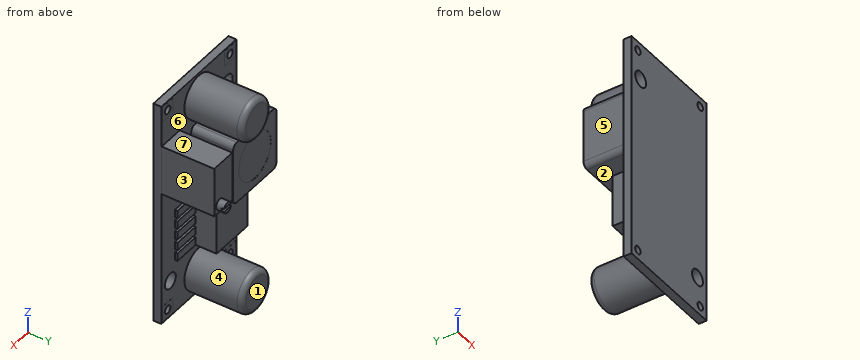
Autodesk Inventor part; units mm, degrees
ref_plane "YZ Plane" through (0, 0, 0) normal (1, 0, 0) x (0, 1, 0)
ref_plane "XZ Plane" through (0, 0, 0) normal (0, 1, 0) x (-1, 0, 0)
ref_plane "XY Plane" through (0, 0, 0) normal (0, 0, 1) x (1, 0, 0)
sketch "Sketch1" plane through (0, 0, 0) normal (0, 1, 0) x (-1, 0, 0)
  line L0 (-10.375, 21.675) -> (10.375, 21.675)
  line L1 (10.375, 21.675) -> (10.375, -21.675)
  line L2 (10.375, -21.675) -> (-10.375, -21.675)
  line L3 (-10.375, -21.675) -> (-10.375, 21.675)
  line L4 (-10.375, 21.675) -> (10.375, -21.675) construction
  line L5 (10.375, 21.675) -> (-10.375, -21.675) construction
  point P0 (0, 0)
  dimension "d0" = 20.75
  dimension "d1" = 43.35
extrude "Extrusion1" add sketch "Sketch1" along normal blind 1.5
sketch "Sketch2" plane through (0, 1.5, 0) normal (0, 1, 0) x (1, 0, 0)
  circle A0 centre (-8.625, -19.925) radius 0.75
  circle A1 centre (-8.625, 19.925) radius 0.75
  circle A2 centre (8.625, -19.925) radius 0.75
  circle A3 centre (8.625, 19.925) radius 0.75
  line L0 (-10.375, -21.675) -> (10.375, -21.675)
  line L1 (10.375, -21.675) -> (10.375, 21.675)
  line L2 (-10.375, 21.675) -> (-10.375, -21.675)
  line L3 (10.375, 21.675) -> (-10.375, 21.675)
  point P0 (0, 0)
  dimension "d4" = 1.5
  dimension "d5" = 1.5
  dimension "d6" = 1.5
  dimension "d7" = 1.5
  dimension "d8" = 1.75
  dimension "d9" = 1.75
  dimension "d10" = 1.75
  dimension "d11" = 1.75
  dimension "d12" = 1.75
  dimension "d13" = 1.75
  dimension "d14" = 1.75
  dimension "d15" = 1.75
extrude "Extrusion2" cut sketch "Sketch2" against normal up to next contours A0 | A1 | A2 | A3
sketch "Sketch3" plane through (0, 1.5, 0) normal (0, 1, 0) x (1, 0, 0)
  circle A0 centre (7.875, 14.675) radius 1.5
  circle A1 centre (-7.875, -14.675) radius 1.5
  line L0 (-10.375, 21.675) -> (-10.375, -21.675)
  line L1 (10.375, 21.675) -> (10.375, -21.675)
  line L2 (10.375, 21.675) -> (-10.375, 21.675)
  line L3 (-10.375, -21.675) -> (10.375, -21.675)
  point P0 (0, 0)
  dimension "d18" = 3
  dimension "d19" = 3
  dimension "d20" = 2.5
  dimension "d21" = 2.5
  dimension "d22" = 7
  dimension "d23" = 7
extrude "Extrusion3" cut sketch "Sketch3" against normal up to next contours A0 | A1
sketch "Sketch4" plane through (0, 1.5, 0) normal (0, 1, 0) x (1, 0, 0)
  line L0 (-7.125, -18.425) -> (-10.125, -18.425)
  line L1 (-10.125, -18.425) -> (-10.125, -21.425)
  line L2 (-10.125, -21.425) -> (-7.125, -21.425)
  line L3 (-7.125, -21.425) -> (-7.125, -18.425)
  circle A0 centre (-8.625, -19.925) radius 0.75
  line L4 (-7.125, -18.425) -> (-10.125, -21.425) construction
  line L5 (-10.125, -18.425) -> (-7.125, -21.425) construction
  line L6 (10.125, -21.425) -> (7.125, -21.425)
  line L7 (7.125, -21.425) -> (7.125, -18.425)
  line L8 (7.125, -18.425) -> (10.125, -18.425)
  line L9 (10.125, -18.425) -> (10.125, -21.425)
  circle A1 centre (8.625, -19.925) radius 0.75
  line L10 (10.125, -21.425) -> (7.125, -18.425) construction
  line L11 (7.125, -21.425) -> (10.125, -18.425) construction
  line L12 (7.125, 18.425) -> (10.125, 18.425)
  line L13 (10.125, 18.425) -> (10.125, 21.425)
  line L14 (10.125, 21.425) -> (7.125, 21.425)
  line L15 (7.125, 21.425) -> (7.125, 18.425)
  circle A2 centre (8.625, 19.925) radius 0.75
  line L16 (7.125, 18.425) -> (10.125, 21.425) construction
  line L17 (10.125, 18.425) -> (7.125, 21.425) construction
  line L18 (-10.125, 21.425) -> (-7.125, 21.425)
  line L19 (-7.125, 21.425) -> (-7.125, 18.425)
  line L20 (-7.125, 18.425) -> (-10.125, 18.425)
  line L21 (-10.125, 18.425) -> (-10.125, 21.425)
  circle A3 centre (-8.625, 19.925) radius 0.75
  line L22 (-10.125, 21.425) -> (-7.125, 18.425) construction
  line L23 (-7.125, 21.425) -> (-10.125, 18.425) construction
  circle A4 centre (-8.625, -19.925) radius 0.75
  circle A5 centre (8.625, -19.925) radius 0.75
  circle A6 centre (-8.625, 19.925) radius 0.75
  circle A7 centre (8.625, 19.925) radius 0.75
  point P0 (0, 0)
  dimension "d26" = 3
  dimension "d27" = 3
  dimension "d28" = 3
  dimension "d29" = 3
  dimension "d30" = 3
  dimension "d31" = 3
  dimension "d32" = 3
  dimension "d33" = 3
extrude "Extrusion4" add sketch "Sketch4" along normal blind 0.01
sketch "Sketch5" plane through (0, 1.5, 0) normal (0, 1, 0) x (1, 0, 0)
  circle A0 centre (0, 17.175) radius 4
  line L0 (10.375, 21.675) -> (-10.375, 21.675)
  point P0 (0, 0)
  dimension "d36" = 8
  dimension "d37" = 4.5
extrude "Extrusion5" add sketch "Sketch5" along normal blind 11
sketch "Sketch6" plane through (0, 1.5, 0) normal (0, 1, 0) x (1, 0, 0)
  circle A0 centre (0, -17.175) radius 4
  line L0 (-10.375, -21.675) -> (10.375, -21.675)
  point P0 (0, 0)
  dimension "d40" = 8
  dimension "d41" = 4.5
extrude "Extrusion6" add sketch "Sketch6" along normal blind 11
sketch "Sketch7" plane through (0, 1.5, 0) normal (0, 1, 0) x (1, 0, 0)
  line L0 (2.125, -12.175) -> (-9.875, -12.175)
  line L1 (-9.875, -12.175) -> (-9.875, -0.175)
  line L2 (-9.875, -0.175) -> (2.125, -0.175)
  line L3 (2.125, -0.175) -> (2.125, -12.175)
  line L4 (2.125, -12.175) -> (-9.875, -0.175) construction
  line L5 (-9.875, -12.175) -> (2.125, -0.175) construction
  line L6 (-10.375, 21.675) -> (-10.375, -21.675)
  circle A0 centre (0, -17.175) radius 4
  point P0 (0, 0)
  point P1 (-3.875, -6.175)
  dimension "d44" = 12
  dimension "d45" = 12
  dimension "d46" = 0.5
  dimension "d47" = 5
extrude "Extrusion7" add sketch "Sketch7" along normal blind 8 contours L0 L1 L2 L3
sketch "Sketch8" plane through (0, 9.5, 0) normal (0, 1, 0) x (1, 0, 0)
  line L0 (2.125, -12.175) -> (-9.875, -12.175)
  line L1 (-9.875, -12.175) -> (2.125, -0.175)
  circle A0 centre (-3.875, -6.175) radius 4.4338
  point P0 (0, 0)
extrude "Extrusion8" cut sketch "Sketch8" against normal blind 0.01
sketch "Sketch9" plane through (0, 1.5, 0) normal (0, 1, 0) x (1, 0, 0)
  line L0 (10.275, -13.675) -> (5.275, -13.675)
  line L1 (5.275, -13.675) -> (5.275, -4.175)
  line L2 (5.275, -4.175) -> (10.275, -4.175)
  line L3 (10.275, -4.175) -> (10.275, -13.675)
  line L4 (10.275, -13.675) -> (5.275, -4.175) construction
  line L5 (5.275, -13.675) -> (10.275, -4.175) construction
  line L6 (-10.375, -21.675) -> (10.375, -21.675)
  line L7 (10.375, 21.675) -> (10.375, -21.675)
  point P0 (0, 0)
  point P1 (7.775, -8.925)
  dimension "d52" = 5
  dimension "d53" = 9.5
  dimension "d54" = 8
  dimension "d55" = 0.1
extrude "Extrusion9" add sketch "Sketch9" along normal blind 10
sketch "Sketch10" plane through (0, 11.5, 0) normal (0, 1, 0) x (1, 0, 0)
  circle A0 centre (8.775, -5.675) radius 1
  line L0 (10.275, -4.175) -> (5.275, -4.175)
  line L1 (10.275, -13.675) -> (10.275, -4.175)
  point P0 (0, 0)
  dimension "d58" = 2
  dimension "d59" = 1.5
  dimension "d60" = 1.5
extrude "Extrusion10" add sketch "Sketch10" along normal blind 1.5
sketch "Sketch11" plane through (8.775, 13, 5.675) normal (0, 1, 0) x (1, 0, 0)
  line L0 (1.224, -0.2665) -> (-1.224, -0.2665)
  line L1 (-1.224, -0.2665) -> (-1.224, 0.2665)
  line L2 (-1.224, 0.2665) -> (1.224, 0.2665)
  line L3 (1.224, 0.2665) -> (1.224, -0.2665)
  line L4 (1.224, -0.2665) -> (-1.224, 0.2665) construction
  line L5 (-1.224, -0.2665) -> (1.224, 0.2665) construction
  point P0 (-8.775, 5.675)
  point P1 (0, 0)
extrude "Extrusion11" cut sketch "Sketch11" against normal blind 0.5
sketch "Sketch12" plane through (0, 1.5, 0) normal (0, 1, 0) x (1, 0, 0)
  line L0 (1.625, 1.325) -> (-6.875, 1.325)
  line L1 (-6.875, 1.325) -> (-6.875, 11.325)
  line L2 (-6.875, 11.325) -> (1.625, 11.325)
  line L3 (1.625, 11.325) -> (1.625, 1.325)
  line L4 (1.625, 1.325) -> (-6.875, 11.325) construction
  line L5 (-6.875, 1.325) -> (1.625, 11.325) construction
  line L6 (-10.375, 21.675) -> (-10.375, -21.675)
  line L7 (2.125, -0.175) -> (-9.875, -0.175)
  point P0 (0, 0)
  point P1 (-2.625, 6.325)
  dimension "d65" = 8.5
  dimension "d66" = 10
  dimension "d67" = 3.5
  dimension "d68" = 1.5
extrude "Extrusion12" add sketch "Sketch12" along normal blind 4.5
sketch "Sketch13" plane through (1.625, 1.5, -1.325) normal (1, 0, 0) x (0, 0, -1)
  line L0 (10, 0) -> (0, 0)
  line L1 (0, 0) -> (1.5, 0)
  line L2 (1.5, 0) -> (1.5, 0.5)
  line L3 (1.5, 0.5) -> (0, 0.5)
  line L4 (0, 0.5) -> (0, 0)
  line L5 (10, 0) -> (8.5, 0)
  line L6 (8.5, 0) -> (8.5, 0.5)
  line L7 (8.5, 0.5) -> (10, 0.5)
  line L8 (10, 0.5) -> (10, 0)
  line L9 (2.12, 0) -> (3.62, 0)
  line L10 (3.62, 0) -> (3.62, 0.5)
  line L11 (3.62, 0.5) -> (2.12, 0.5)
  line L12 (2.12, 0.5) -> (2.12, 0)
  line L13 (6.38, 0) -> (7.88, 0)
  line L14 (7.88, 0) -> (7.88, 0.5)
  line L15 (7.88, 0.5) -> (6.38, 0.5)
  line L16 (6.38, 0.5) -> (6.38, 0)
  line L17 (4.24, 0) -> (5.74, 0)
  line L18 (5.74, 0) -> (5.74, 0.5)
  line L19 (5.74, 0.5) -> (4.24, 0.5)
  line L20 (4.24, 0.5) -> (4.24, 0)
  point P0 (-1.325, -1.5)
  dimension "d71" = 1.5
  dimension "d72" = 0.5
  dimension "d73" = 1.5
  dimension "d74" = 0.5
  dimension "d75" = 1.5
  dimension "d76" = 1.5
  dimension "d77" = 0.5
  dimension "d78" = 0.62
  dimension "d79" = 0.62
  dimension "d80" = 1.5
  dimension "d81" = 0.62
extrude "Extrusion13" add sketch "Sketch13" along normal blind 5
fillet "Fillet1" radius 1 6 edges at (2.125, 5.5, 12.175) (2.125, 5.5, 0.175) (-9.875, 5.5, 12.175) (-9.875, 5.5, 0.175) (-4, 12.5, 17.175) (-4, 12.5, -17.175)
properties part number "pcb_with_elements"
Geometry check sheet. Reference: the model listing, model coordinates, mm. Face numbers are marked on the shaded views. A direction names the side the tool comes from. Give positions to 0.01 mm unless a question says otherwise; leave off trailing zeros. Loops run counter-clockwise (first coordinate to the right, second up) from the corner with the lowest first, then second, coordinate; pieces in that order, holes last. Notation, with made-up numbers: (81, 38) - (107, 38) arc R19 ccw to (107, 66) - close; hole circle Ø9 at (59, 81). An arc over 180 degrees is marked (long way). Use CSV: the item, a comma, the result in double quotes. Start each with the question number.
Q1. Scan lines: probe 1 along X at (y, z) = (5.5, 11) (3 decimals); probe 2 along Z at (x, y) = (1.5, 4.75) (3 decimals); probe 3 along X at (y, z) = (4.75, -3.5) (3 decimals). Record each from-to range of solid material in increasing order. Write a range as from..to.
Q2. Access from +Z, -Z, +X, -X, +Y, -Y to the whole of each face (thin tool, end or side, straight path). Record for the marked faces 1, 2, 3 and 4.
Q3. Go/stop test with flat-tipped pins: pin 1 Ø0.8 at (x, z) = (3.5, -10.5) entering from +Y; pin 2 Ø3 at (x, y) = (3.5, 11.5) entering from +Z; pin 3 Ø1.5 at (x, y) = (6.5, 9) entering from -Z (3 decimals). Record where each tip stops, or that it passes through.
Q4. Section check B-B, the plane y = 8.5. Record the cut outline in (x, z) (3 decimals).
Q5. Section check D-D, the plane x = 0. Record the cut outline in (y, z) (3 decimals), and give its area (3 significant figures).
Q6. Section check C-C, the plane y = 2.5. Record the cut outline in (x, z) (3 decimals), and give its area (3 significant figures).
Q7. Release check for a two-part mould opening along Z. For the marked faces 5, 6 and 7 record: +Z half, -Z half, draft (parallel to the pull), parting line (faces both ways), or undercut.
Q8. Section check A-A, the plane z = -4.5. Record the cut outline in (x, y) (3 decimals).
Findings below:
1,probe 1,"x = -9.875..2.125, 5.275..10.275"
1,probe 2,"z = -20.883..-13.467, -11.325..-1.325, 0.248..12.102, 13.467..20.883"
1,probe 3,"x = -6.875..1.625"
2,face 1,"+Z, -Z, +X, -X, +Y"
2,face 2,"+X, -X, +Y"
2,face 3,"+Z, -Z, +X, +Y"
2,face 4,"+Y"
3,pin 1,"stops at y = 2"
3,pin 2,"stops at z = 20.64"
3,pin 3,"stops at z = 4.175"
4,outline,"(-9.875, 1.175) arc R1 ccw to (-8.875, 0.175) - (1.125, 0.175) arc R1 ccw to (2.125, 1.175) - (2.125, 11.175) arc R1 ccw to (1.125, 12.175) - (-8.875, 12.175) arc R1 ccw to (-9.875, 11.175) - close; circle Ø8 at (0, -17.175); circle Ø8 at (0, 17.175); (5.275, 4.175) - (10.275, 4.175) - (10.275, 13.675) - (5.275, 13.675) - close"
5,outline,"(0, -21.675) - (1.5, -21.675) - (1.5, -21.175) - (11.5, -21.175) arc R1 ccw to (12.5, -20.175) - (12.5, -14.175) arc R1 ccw to (11.5, -13.175) - (1.5, -13.175) - (1.5, -11.325) - (6, -11.325) - (6, -1.325) - (1.5, -1.325) - (1.5, 0.175) - (9.5, 0.175) - (9.5, 4.02) - (9.49, 4.02) - (9.49, 8.33) - (9.5, 8.33) - (9.5, 12.175) - (1.5, 12.175) - (1.5, 13.175) - (11.5, 13.175) arc R1 ccw to (12.5, 14.175) - (12.5, 20.175) arc R1 ccw to (11.5, 21.175) - (1.5, 21.175) - (1.5, 21.675) - (0, 21.675) - close"
5,area,"381 mm^2"
6,outline,"(-9.875, 1.175) arc R1 ccw to (-8.875, 0.175) - (1.125, 0.175) arc R1 ccw to (2.125, 1.175) - (2.125, 11.175) arc R1 ccw to (1.125, 12.175) - (-8.875, 12.175) arc R1 ccw to (-9.875, 11.175) - close; (-6.875, -11.325) - (1.625, -11.325) - (1.625, -1.325) - (-6.875, -1.325) - close; circle Ø8 at (0, -17.175); circle Ø8 at (0, 17.175); (5.275, 4.175) - (10.275, 4.175) - (10.275, 13.675) - (5.275, 13.675) - close"
6,area,"376 mm^2"
7,face 5,"draft"
7,face 6,"undercut"
7,face 7,"+Z half"
8,outline,"(-10.375, 0) - (10.375, 0) - (10.375, 1.5) - (6.625, 1.5) - (6.625, 2) - (1.625, 2) - (1.625, 6) - (-6.875, 6) - (-6.875, 1.5) - (-10.375, 1.5) - close"
